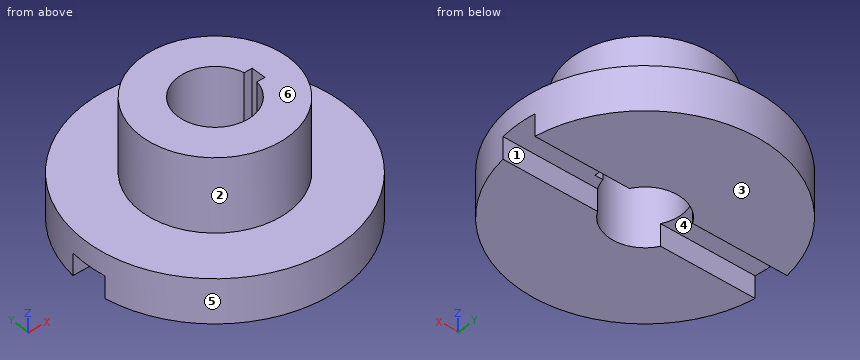
```python
from build123d import *

# Parameters (mm, degrees)
SKETCH1_R           = 175
BOSS_EXTRUDE1_DEPTH = 60
SKETCH2_R           = 100
BOSS_EXTRUDE2_DEPTH = 100
CUT_EXTRUDE1_DEPTH  = 30
CUT_EXTRUDE2_DEPTH  = 295.703240566


with BuildPart() as part:
    # Sketch1 → Boss-Extrude1 (new body)
    with BuildSketch(Plane.XY):
        Circle(SKETCH1_R)
    extrude(amount=BOSS_EXTRUDE1_DEPTH)

    # Sketch2 → Boss-Extrude2 (add)
    with BuildSketch(Plane.XY.offset(60)):
        Circle(SKETCH2_R)
    extrude(amount=BOSS_EXTRUDE2_DEPTH)

    # Sketch4 → Cut-Extrude1 (cut)
    with BuildSketch(Plane.XY):
        with BuildLine():
            Line((173.205080757, 25), (-173.205080757, 25))
            ThreePointArc((-173.205080757, 25), (-175, 0), (-173.205080757, -25))
            Line((-173.205080757, -25), (173.205080757, -25))
            ThreePointArc((173.205080757, -25), (175, 0), (173.205080757, 25))
        make_face()
    extrude(amount=CUT_EXTRUDE1_DEPTH, mode=Mode.SUBTRACT)

    # Sketch6 → Cut-Extrude2 (cut, through all)
    with BuildSketch(Plane.XY.offset(160)):
        with BuildLine():
            Line((59.999794856, 10), (59.999794856, -10))
            Line((59.999794856, -10), (48.989794856, -10))
            ThreePointArc((48.989794856, -10), (-50, 0), (48.989794856, 10))
            Line((48.989794856, 10), (59.999794856, 10))
        make_face()
    extrude(amount=-CUT_EXTRUDE2_DEPTH, mode=Mode.SUBTRACT)


solid = part.part
```
Build history of the part. All positions in model axes, mm. Face numbers are marked on the shaded views. A direction names the side the tool comes from. Coordinates: 2 decimals unless noted, no trailing zeros. Write each loop counter-clockwise with the first axis right and the second up, starting at its lowest first coordinate (ties: lowest second). Pieces come first, ordered by that corner, then holes.
1. Band-saw the part on D-D, the plane y = 59. Give the cut face in (x, z), and give its area (3 significant figures).
Answer block:
outline: (-164.75, 0) - (164.75, 0) - (164.75, 60) - (80.74, 60) - (80.74, 160) - (-80.74, 160) - (-80.74, 60) - (-164.75, 60) - close
area: 35,900 mm2
2. 3-axis set-ups, long thin cutter, end or side, ignore diameter. For the marked faces 1, 2 and 3: which of +Z, -Z, +X, -X, +Y, -Y reach the whole face in a straight line?
Answer block:
face 1: -Z, +X, -X
face 2: +Z
face 3: -Z, +X, -X, +Y, -Y
3. Band-saw the part on A-A, the plane x = 0. Give the cut face in (y, z), and give its area (3 significant figures).
Answer block:
outline: (-175, 0) - (-50, 0) - (-50, 160) - (-100, 160) - (-100, 60) - (-175, 60) - close; (50, 0) - (175, 0) - (175, 60) - (100, 60) - (100, 160) - (50, 160) - close
area: 25,000 mm2
4. Pull direction Y, two halves, no side cores. Call the marked faces 4, 5 and 6: released by +Y, released by -Y, zero draft, split by the parting line, or undercut.
Answer block:
face 4: undercut
face 5: split by the parting line
face 6: zero draft
5. Band-saw the part on C-C, the plane z = 40. Give the cut face in (x, y).
Answer block:
outline: circle Ø350 at (0, 0); hole (48.99, -10) - (60, -10) - (60, 10) - (48.99, 10) arc R50 ccw (long way) to start
6. Drop flat-ended pins along their axis: pin 1 (1.5 mm diameter, centred on y = 123, z = 40.5, fed in from -X); pin 2 (24 mm diameter, centred on x = 134, z = 10, fed in from -Y); pin 3 (5 mm diameter, centred on x = -75, z = 88.5, fed in from +Y). Give the stop position or say it passes through.
Answer block:
pin 1: stops at x = -125.22
pin 2: stops at y = -125.46
pin 3: stops at y = 68.87
7. Band-saw the part on B-B, the plane y = 0. Give the cut face in (x, z), and give its area (3 significant figures).
Answer block:
outline: (-175, 30) - (-50, 30) - (-50, 160) - (-100, 160) - (-100, 60) - (-175, 60) - close; (60, 30) - (175, 30) - (175, 60) - (100, 60) - (100, 160) - (60, 160) - close
area: 16,200 mm2
8. Drill centre lines: probe 1 along Y at (x, z) = (0, 126); probe 2 along Z at (x, y) = (-110.5, -124.5); probe 3 along Y at (x, z) = (3.5, 14) (3 decimals). Where is each one in solid material? Low to high.
Answer block:
probe 1: y = -100 to -50, 50 to 100
probe 2: z = 0 to 60
probe 3: y = -174.965 to -49.877, 49.877 to 174.965
